from build123d import *

# Parameters (mm, degrees)
F0_W     = 42
F0_H     = 10
F1_DEPTH = 27
F2_R     = 1.7
F3_DEPTH = 27.001
F4_W     = 13.5
F4_H     = 5.9
F5_DEPTH = 4
F4_R     = 2.2
F6_DEPTH = 25
F7_R     = 4.2
F8_DEPTH = 3
F9_R     = 1.99999


# Not quite as in the source:
# - a fillet or chamfer is up to 0.001 mm smaller than in the source, because OpenCascade refuses the exact size


with BuildPart() as f1:
    # F0 (on Top) → F1 (new body)
    with BuildSketch(Plane.XY):
        with Locations((4.146153807, 5)):
            Rectangle(F0_W, F0_H)
    extrude(amount=F1_DEPTH)

    # F2 (on face) → F3 (cut, through all)
    with BuildSketch(Plane.XY.offset(27)):
        with BuildLine():
            ThreePointArc((-13.053846193, 5), (-11.353846193, 3.3), (-9.653846193, 5))
            ThreePointArc((-9.653846193, 5), (-11.353846193, 6.7), (-13.053846193, 5))
        make_face()
        with Locations((19.646153807, 5)):
            Circle(F2_R)
    extrude(amount=-F3_DEPTH, mode=Mode.SUBTRACT)

    # F4 (on face) → F5 (join)
    with BuildSketch(Plane(origin=(0, 10, 0), x_dir=(-1, 0, 0), z_dir=(0, 1, 0))):
        with Locations((-18.396153807, 17)):
            Rectangle(F4_W, F4_H)
        with Locations((10.103846193, 17)):
            Rectangle(F4_W, F4_H)
    extrude(amount=F5_DEPTH)

    # F4 (on face) → F6 (cut)
    with BuildSketch(Plane(origin=(0, 10, 0), x_dir=(-1, 0, 0), z_dir=(0, 1, 0))):
        with Locations((-4.146153807, 17)):
            Circle(F4_R)
    extrude(amount=-F6_DEPTH, mode=Mode.SUBTRACT)

    # F7 (on face) → F8 (cut)
    with BuildSketch(Plane.XZ):
        with Locations((4.146153807, 17)):
            Circle(F7_R)
    extrude(amount=-F8_DEPTH, mode=Mode.SUBTRACT)

    # F9 (radius 2 in the source; OpenCascade refuses exactly that, so slightly less here)
    f9_edges = [f1.edges().sort_by_distance(p)[0] for p in [
        (-0.053846, 3, 17),
    ]]
    fillet(f9_edges, radius=F9_R)


solid = f1.part
The listing builds one solid part. Answer for the finished solid, in the listing's coordinates (mm). A direction names the side the tool comes from. Coordinates: 2 decimals unless noted, no trailing zeros. Loops run counter-clockwise (first coordinate to the right, second up) from the corner with the lowest first, then second, coordinate; pieces in that order, holes last. Notation, with made-up numbers: (83, 53.25) -> (118, 53.25) arc R20 ccw to (118, 75.25) -> close; hole circle Ø1 at (40.25, -40). An arc over 180 degrees is marked (long way). Answer in a Markdown table with one row per item. Add a question column.
1. The part is cut by section D-D, the plane x = 12.5. Write down the section's boundary in (y, z), then the cut area to 3 significant figures.
2. Consider line 1 (X direction, y = 4, z = 8.25); line 2 (Y direction, x = -9, z = 7); line 3 (Z direction, x = 5, y = 2.75). Determine where each line is inside the solid, lowest interval first. Write a range as [from, to].
3. The part is cut by section B-B, the plane z = 17. Count the separate pieces of the cut face and the enclosed holes in it, then the cut area to 3 significant figures.
4. Determine the mould class of faces 1 (the flat face through (-16.854, 5, 13)), 2 (the cylindrical face through (-9.783, 4.349, 13.689)), 3 (the flat face through (-10, 12, 14.05)), 4 (the flat face through (25.146, 5, 13)) for opening direction X: +X half, -X half, draft (parallel to the pull), parting line (faces both ways), or undercut.
5. Flat-ended cylindrical pins translate along their axes: P1, Ø13.5, axis at x = 4.15, z = 17, coming from the +Y side; P2, Ø2, axis at x = 3.5, z = 16.5, coming from the -Y side; P3, Ø1.5, axis at x = -10, y = 12.5, coming from the +Z side; P4, Ø1.2, axis at x = 17, y = 12.5, coming from the -Z side. Find the tip coordinate at first contact, or state that the pin passes through.
6. The part is cut by section A-A, the plane y = 5. Write down the section's boundary in (x, z), then the cut area to 3 significant figures.
7. The part is cut by section C-C, the plane z = 8. Write down the section's boundary in (x, y).
8. For faces 5 (the cylindrical face through (3.599, 0.493, 21.164)), 6 (the flat face through (-3.354, 12, 17)), 7 (the flat face through (18, 12, 14.05)), determine the directions among +Z, -Z, +X, -X, +Y, -Y from which every point of the face is accessible in a straight line to the end or side of a thin tool.
Answer below:
| question | item | result |
|---|---|---|
| 1 | outline | (0, 0) -> (10, 0) -> (10, 14.05) -> (14, 14.05) -> (14, 19.95) -> (10, 19.95) -> (10, 27) -> (0, 27) -> close |
| 1 | area | 294 mm2 |
| 2 | line 1 | [-16.85, -12.73], [-9.98, 18.27], [21.02, 25.15] |
| 2 | line 2 | [0, 10] |
| 2 | line 3 | [0, 13.95], [20.05, 27] |
| 3 | separate pieces | 2 |
| 3 | enclosed holes | 2 |
| 3 | area | 456 mm2 |
| 4 | face 1 | -X half |
| 4 | face 2 | undercut |
| 4 | face 3 | draft |
| 4 | face 4 | +X half |
| 5 | P1 | y = 10 |
| 5 | P2 | through |
| 5 | P3 | z = 19.95 |
| 5 | P4 | z = 14.05 |
| 6 | outline | (-16.85, 0) -> (-13.05, 0) -> (-13.05, 27) -> (-16.85, 27) -> close; (-9.65, 0) -> (17.95, 0) -> (17.95, 27) -> (-9.65, 27) -> close; (21.35, 0) -> (25.15, 0) -> (25.15, 27) -> (21.35, 27) -> close; hole circle Ø4.4 at (4.15, 17) |
| 6 | area | 935 mm2 |
| 7 | outline | (-16.85, 0) -> (25.15, 0) -> (25.15, 10) -> (-16.85, 10) -> close; hole circle Ø3.4 at (-11.35, 5); hole circle Ø3.4 at (19.65, 5) |
| 8 | face 5 | -Y |
| 8 | face 6 | +Z, -Z, +Y |
| 8 | face 7 | -Z, +X, -X, +Y |
